Geometry check sheet. Reference: the model listing, model coordinates, mm. A direction names the side the tool comes from. Coordinates: 2 decimals unless noted, no trailing zeros. Order: outer loops, then holes, each group sorted by start corner. A loop starts at its lowest first (then second) coordinate and runs counter-clockwise, first axis right, second up. Notation, with made-up numbers: M 20.25,-8 L 32.25,-8 A22 cw 32.25,20 Z; hole C -21,55 d10. An arc over 180 degrees is marked long. One line per item, written item: value. Start each with the question number.
1) Go/stop test with flat-tipped pins: P1, Ø0.8, axis at x = 414, y = 19, coming from the +Z side; P2, Ø1.9, axis at x = 329.5, z = 14, coming from the +Y side; P3, Ø0.7, axis at x = 233, y = -19.5, coming from the -Z side; P4, Ø5, axis at y = -10, z = -8, coming from the +X side. Record where each tip stops, or that it passes through.
2) Sectioned sample at B-B, the plane z = -7. State how many separate pieces and enclosed holes the cut face has, then the cut area to 3 significant figures.
3) Access from +Z, -Z, +X, -X, +Y, -Y to the whole of each face (thin tool, end or side, straight path). Record for faces 1 (the flat face through (295.8, -8.614, -6.974)), 2 (the flat face through (296, 0, 3.784)), 3 (the flat face through (0, 0, -3)).
4) Thickness scan on L1, parallel to Y at x = 284, z = 10; L2, parallel to Z at x = 257, y = 12.5; L3, parallel to Z at x = 193, y = 14.5. Record the ranges inside material, lowest first. Write a range as from..to.
5) Sectioned sample at A-A, the plane y = -0.5. Enter the section's corners in (x, z).
```python
from build123d import *

# Parameters (mm, degrees)
F1_DEPTH = 600


with BuildPart() as f1:
    # F0 (on Right) → F1 (new body)
    with BuildSketch(Plane.YZ):
        Polygon((-19.76107, 15.892943), (-22.115579, 15.892943), (-26.824599, 12.192998), (-26.824599, -15.892943), (-25.926842, -15.892943), (-24.826841, 1.698052), (-23.326841, 1.698052), (-22.926842, -15.892943), (-21.428242, -15.892943), (-20.329641, 1.698052), (-18.83157, 1.698052), (-17.527344, -15.892943), (-15.748855, -15.892943), (-14.859609, 1.698052), (-13.318252, 1.698052), (-12.547573, -15.892943), (-11.30263, -15.892943), (-10.16482, 1.698052), (-9.227727, 1.698052), (-7.982784, -15.892943), (7.982784, -15.892943), (9.227727, 1.698052), (10.16482, 1.698052), (11.30263, -15.892943), (12.547573, -15.892943), (13.318252, 1.698052), (14.859609, 1.698052), (15.748855, -15.892943), (17.527344, -15.892943), (18.83157, 1.698052), (20.329641, 1.698052), (21.428242, -15.892943), (22.926842, -15.892943), (23.326841, 1.698052), (24.826841, 1.698052), (25.926842, -15.892943), (26.824599, -15.892943), (26.824599, 12.192998), (22.115579, 15.892943), (19.76107, 15.892943), (19.76107, 12.024819), (18.247455, 12.024819), (18.247455, 3.784032), (0, 3.784032), (-18.247455, 3.784032), (-18.247455, 12.024819), (-19.76107, 12.024819), align=None)
    extrude(amount=F1_DEPTH)


solid = f1.part
```
Final values:
1. P1: stops at z = 12.02
1. P2: stops at y = 25.73
1. P3: stops at z = 1.7
1. P4: stops at x = 600
2. separate pieces: 9
2. enclosed holes: 0
2. area: 20,900 mm^2
3. face 1: -Z, +X, -X
3. face 2: +Z, +X, -X
3. face 3: +Z, -Z, -X, +Y, -Y
4. L1: y = -26.82..-18.25, 18.25..26.82
4. L2: z = -15.89..3.78
4. L3: z = 1.7..3.78
5. outline: M 0,-15.89 L 600,-15.89 L 600,3.78 L 0,3.78 Z
